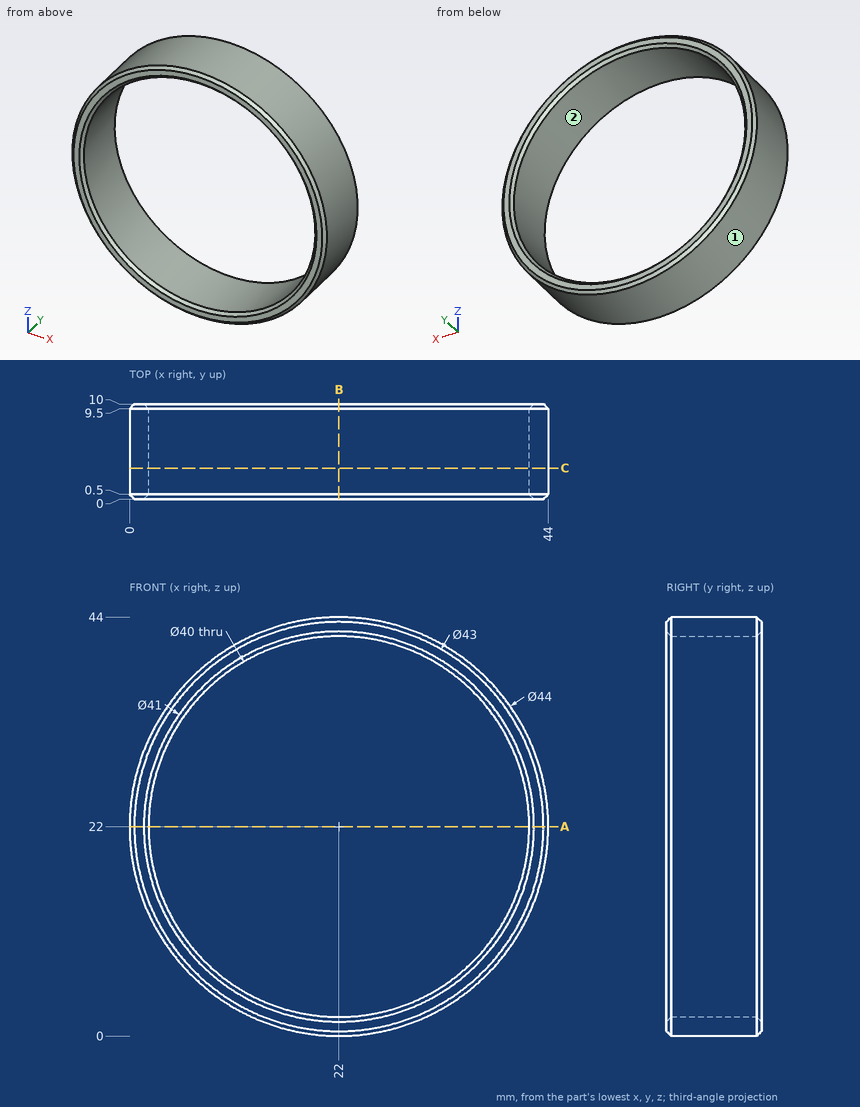
Geometry check sheet. Reference: drawing and pictorial views, mm from the part's lowest x, y, z. Round coordinates to 2 decimals unless told otherwise and drop trailing zeros. Loops run counter-clockwise (first coordinate to the right, second up) from the corner with the lowest first, then second, coordinate; pieces in that order, holes last. Notation, with made-up numbers: (86, 45.25) - (129, 45.25) arc R35 cw to (129, 78.25) - close; hole circle Ø1 at (-7, 54). An arc over 180 degrees is marked (long way). One line per question, with ' | ' between items. Start each with the question number.
1. Scan lines: line 1 (X direction, y = 5.5, z = 22); line 2 (Z direction, x = 30, y = 8.5). Record each from-to range of solid material in increasing order. Write a range as [from, to].
2. Cross-section at B-B on x = 22. Record the cut outline in (y, z).
3. Cross-section at C-C on y = 3.25. Record the cut outline in (x, z).
4. Draft check along Z on the marked faces 1 and 2. Enter one of: released by +Z, released by -Z, zero draft, split by the parting line, or undercut.
5. Depth check by flat-ended pin: pin 1 (3 mm diameter, centred on x = 34.5, y = 3, fed in from -Z); pin 2 (6 mm diameter, centred on y = 2.5, z = 5.5, fed in from -X); pin 3 (5 mm diameter, centred on y = 3.5, z = 31.5, fed in from +X); pin 4 (10 mm diameter, centred on x = 21, z = 12, fed in from +Y). Enter the tip coordinate at first touch or a pass-through.
6. Cross-section at A-A on z = 22. Record the cut outline in (x, y).
Taken from the geometry:
1) line 1: [0, 2], [42, 44] | line 2: [1.51, 3.67], [40.33, 42.49]
2) outline: (0, 0.5) - (0.5, 0) - (9.5, 0) - (10, 0.5) - (10, 1.5) - (9.5, 2) - (0.5, 2) - (0, 1.5) - close; (0, 42.5) - (0.5, 42) - (9.5, 42) - (10, 42.5) - (10, 43.5) - (9.5, 44) - (0.5, 44) - (0, 43.5) - close
3) outline: circle Ø44 at (22, 22); hole circle Ø40 at (22, 22)
4) face 1: split by the parting line | face 2: undercut
5) pin 1: z = 2.95 | pin 2: x = 4.63 | pin 3: x = 42.86 | pin 4: through
6) outline: (0, 0.5) - (0.5, 0) - (1.5, 0) - (2, 0.5) - (2, 9.5) - (1.5, 10) - (0.5, 10) - (0, 9.5) - close; (42, 0.5) - (42.5, 0) - (43.5, 0) - (44, 0.5) - (44, 9.5) - (43.5, 10) - (42.5, 10) - (42, 9.5) - close
